```python
from build123d import *

# Parameters (mm, degrees)
BOSS_EXTRUDE1_DEPTH     = 5
CUT_EXTRUDE1_DEPTH      = 92.215662378
CUT_EXTRUDE1_DEPTH_BACK = 92.215662378
SKETCH2_R               = 2.75
CUT_EXTRUDE2_DEPTH      = 92.215662378
CUT_EXTRUDE2_DEPTH_BACK = 92.215662378
CHAMFER3_SIZE           = 2
CUT_EXTRUDE3_DEPTH      = 90.804241831
CUT_EXTRUDE3_DEPTH_BACK = 90.804241831
SKETCH4_W               = 120
SKETCH4_H               = 35
CHAMFER4_SIZE           = 2
SKETCH5_R               = 5
CUT_EXTRUDE4_DEPTH      = 3


with BuildPart() as part:
    # Sketch1 → Boss-Extrude1 (new body)
    with BuildSketch(Plane(origin=(0, 0, 0), x_dir=(1, 0, 0), z_dir=(0, 1, 0))):
        Polygon((-73.8, 35.677122405), (-83.8, 35.677122405), (-83.8, -35.677122405), (-73.8, -35.677122405), (73.8, -35.677122405), (83.8, -35.677122405), (83.8, 35.677122405), (73.8, 35.677122405), align=None)
    extrude(amount=BOSS_EXTRUDE1_DEPTH)

    # Sketch2 → Cut-Extrude1 (cut, two sides: drawn at the far end of the back side and taken through both)
    with BuildSketch(Plane(origin=(0, 5, 0), x_dir=(1, 0, 0), z_dir=(0, 1, 0)).offset(-CUT_EXTRUDE1_DEPTH_BACK)):
        with Locations(Location((-73.8, -15.5, 0), (0, 0, 270))):
            Circle(SKETCH2_R)
        with Locations(Location((-73.8, 15.5, 0), (0, 0, 270))):
            Circle(SKETCH2_R)
        with Locations(Location((73.797239672, -20, 0), (0, 0, 270))):
            Circle(SKETCH2_R)
        with Locations(Location((73.797239672, 20, 0), (0, 0, 270))):
            Circle(SKETCH2_R)
    extrude(amount=CUT_EXTRUDE1_DEPTH + CUT_EXTRUDE1_DEPTH_BACK, mode=Mode.SUBTRACT)

    # Sketch3 → Cut-Extrude2 (cut, two sides: drawn at the far end of the back side and taken through both)
    with BuildSketch(Plane(origin=(0, 5, 0), x_dir=(1, 0, 0), z_dir=(0, 1, 0)).offset(-CUT_EXTRUDE2_DEPTH_BACK)):
        Polygon((-63.8, -22.5), (53.754373535, -24.93027399), (90.089947098, -33.354383806), (45.106765394, -114.519737278), (-93.808894925, -48.481732373), (-93.808894925, -22.5), align=None)
        Polygon((53.754373535, 24.93027399), (-63.8, 22.5), (-93.808894925, 22.5), (-93.808894925, 75.103676807), (90.089947098, 109.537779365), (90.089947098, 33.354383806), align=None)
    extrude(amount=CUT_EXTRUDE2_DEPTH + CUT_EXTRUDE2_DEPTH_BACK, mode=Mode.SUBTRACT)

    # Chamfer3
    # the kernel refuses this chamfer: 2 mm, written as the material it takes off along each edge
    with BuildSketch(Plane(origin=(83.8, 0, 37.039476252), x_dir=(-0.9996219169112968, -0.027495876610586292, 0), z_dir=(0, 0, -1))) as chamfer3_piece_1:
        Polygon((CHAMFER3_SIZE * 0.999621916911, CHAMFER3_SIZE * 0.0274958766106), (-CHAMFER3_SIZE * 0.0274958766106, CHAMFER3_SIZE * 0.999621916911), (0, 0), align=None)
    extrude(amount=74.078952505, mode=Mode.SUBTRACT)
    with BuildSketch(Plane(origin=(58.89664073, 0, 25.036583248), x_dir=(0.020661384909083567, -0.027495876610586414, -0.9994083669566981), z_dir=(-0.9997863692752371, 0, -0.020669199583903272))) as chamfer3_piece_2_section:
        Polygon((CHAMFER3_SIZE * 0.999621916911, -CHAMFER3_SIZE * 0.0274958766106), (-CHAMFER3_SIZE * 0.0274958766106, -CHAMFER3_SIZE * 0.999621916911), (0, 0), align=None)
    chamfer3_piece_2 = extrude(amount=127.866224079, mode=Mode.PRIVATE)
    chamfer3_piece_2 = split(chamfer3_piece_2, bisect_by=Plane(origin=(6.389506061, 0.738517017, 22.5), z_dir=(0, 0, 1)), keep=Keep.TOP, mode=Mode.PRIVATE)
    chamfer3_piece_2 = split(chamfer3_piece_2, bisect_by=Plane(origin=(8.475011093, 0.738517017, 14.432618822), z_dir=(-0.22585154444898248, 0, 0.9741617318854243)), keep=Keep.TOP, mode=Mode.PRIVATE)
    add(chamfer3_piece_2, mode=Mode.SUBTRACT)
    with BuildSketch(Plane(origin=(-68.942267195, 0, -22.393690742), x_dir=(0.020661384909228912, -0.027495876610586358, 0.9994083669566951), z_dir=(0.9997863692752341, 0, -0.02066919958404867))) as chamfer3_piece_3_section:
        Polygon((CHAMFER3_SIZE * 0.999621916911, -CHAMFER3_SIZE * 0.0274958766106), (-CHAMFER3_SIZE * 0.0274958766106, -CHAMFER3_SIZE * 0.999621916911), (0, 0), align=None)
    chamfer3_piece_3 = extrude(amount=127.866224079, mode=Mode.PRIVATE)
    chamfer3_piece_3 = split(chamfer3_piece_3, bisect_by=Plane(origin=(6.389506061, 0.738517017, -22.5), z_dir=(0, 0, -1)), keep=Keep.TOP, mode=Mode.PRIVATE)
    chamfer3_piece_3 = split(chamfer3_piece_3, bisect_by=Plane(origin=(8.475011093, 0.738517017, -14.432618822), z_dir=(-0.22585154444898248, 0, -0.9741617318854243)), keep=Keep.TOP, mode=Mode.PRIVATE)
    add(chamfer3_piece_3, mode=Mode.SUBTRACT)

    # Sketch4 → Cut-Extrude3 (cut, two sides: drawn at the far end of the back side and taken through both)
    with BuildSketch(Plane.XZ.offset(-CUT_EXTRUDE3_DEPTH_BACK)):
        Rectangle(SKETCH4_W, SKETCH4_H)
    extrude(amount=CUT_EXTRUDE3_DEPTH + CUT_EXTRUDE3_DEPTH_BACK, mode=Mode.SUBTRACT)

    # Chamfer4
    chamfer4_edges = [part.edges().sort_by_distance(p)[0] for p in [
        (0, 0, -17.5),
        (60, 0, 0),
        (0, 0, 17.5),
        (-60, 0, 0),
    ]]
    chamfer(chamfer4_edges, length=CHAMFER4_SIZE)

    # Sketch5 → Cut-Extrude4 (cut)
    with BuildSketch(Plane.XZ):
        with Locations(Location((-73.8, 15.5, 0), (0, 0, 270))):
            Circle(SKETCH5_R)
        with Locations(Location((-73.8, -15.5, 0), (0, 0, 270))):
            Circle(SKETCH5_R)
        with Locations(Location((73.797239672, 20, 0), (0, 0, 270))):
            Circle(SKETCH5_R)
        with Locations(Location((73.797239672, -20, 0), (0, 0, 270))):
            Circle(SKETCH5_R)
    extrude(amount=-CUT_EXTRUDE4_DEPTH, mode=Mode.SUBTRACT)


solid = part.part
```
The model under review builds one solid part; all positions refer to its coordinate system, in mm. A direction names the side the tool comes from. Round coordinates to 2 decimals unless told otherwise and drop trailing zeros. Loops run counter-clockwise (first coordinate to the right, second up) from the corner with the lowest first, then second, coordinate; pieces in that order, holes last. Notation, with made-up numbers: M 1,19.25 L 25,19.25 A12 cw 25,32.25 Z; hole C 28.5,-8.75 d7. An arc over 180 degrees is marked long. Put each result on its own line as item: value.
Q1. Consider section A-A, the plane z = 4.5. Give the boundary of the cut face in (x, y).
Result set:
outline: M -83.8,0 L -62,0 L -60,2 L -60,5 L -83.8,5 Z; M 60,2 L 62,0 L 81.8,0 L 83.8,2 L 83.8,5 L 60,5 Z
Q2. Machinability: for faces 4 (the flat face through (-51, 1, -22.5)), 5 (the cylindrical face through (68.916, 1.479, -18.916)), 6 (the flat face through (60, 4, 0)), which of the approach directions +Z, -Z, +X, -X, +Y, -Y give a long, thin tool a straight path to every point of the face, cutting with its end or side? Answer none if there is none.
Result set:
face 4: -Z, -X, -Y
face 5: -Y
face 6: +Y, -Y
Q3. Consider section C-C, the plane x = -73.8. Give the boundary of the cut face in (y, z), then the cut area to 3 significant figures.
Result set:
outline: M 0,-22.5 L 5,-22.5 L 5,-18.25 L 3,-18.25 L 3,-20.5 L 0,-20.5 Z; M 0,-10.5 L 3,-10.5 L 3,-12.75 L 5,-12.75 L 5,12.75 L 3,12.75 L 3,10.5 L 0,10.5 Z; M 0,20.5 L 3,20.5 L 3,18.25 L 5,18.25 L 5,22.5 L 0,22.5 Z
area: 143 mm²
Q4. Consider section D-D, the plane x = -37. Give the boundary of the cut face in (y, z).
Result set:
outline: M 0,-22.5 L 1.45,-22.5 L 2,-23.05 L 5,-23.05 L 5,-17.5 L 2,-17.5 L 0,-19.5 Z; M 0,19.5 L 2,17.5 L 5,17.5 L 5,23.05 L 2,23.05 L 1.45,22.5 L 0,22.5 Z
Q5. To check wall thickness, follow L1, parallel to X at y = 3.15, z = -7; L2, parallel to Z at x = 73, y = 1.3; L3, parallel to X at y = 2.5, z = -16.5. State the ranges of each line that lie inside material, in increasing order.
Result set:
L1: x = -83.8 to -60, 60 to 83.8
L2: z = -29.39 to -24.94, -15.06 to 15.06, 24.94 to 29.39
L3: x = -83.8 to -78.7, -68.9 to -60, 60 to 70.23, 77.37 to 83.8
Q6. Consider section B-B, the plane x = -13. Give the boundary of the cut face in (y, z), then the cut area to 3 significant figures.
Result set:
outline: M 0,-22.5 L 0.95,-22.5 L 2,-23.55 L 5,-23.55 L 5,-17.5 L 2,-17.5 L 0,-19.5 Z; M 0,19.5 L 2,17.5 L 5,17.5 L 5,23.55 L 2,23.55 L 0.95,22.5 L 0,22.5 Z
area: 53.4 mm²
Q7. For pin 1 (3 mm diameter, centred on x = 74, z = -22.5, fed in from -Y); pin 2 (6 mm diameter, centred on x = 73.8, z = -20, fed in from +Y); pin 3 (1.5 mm diameter, centred on x = 26.5, y = 4, fed in from +Z); pin 4 (4.5 mm diameter, centred on x = -73.8, z = 15.5, fed in from +Y), all flat-tipped, find the tip position at first contact; note any pin that passes through.
Result set:
pin 1: stops at y = 3
pin 2: stops at y = 5
pin 3: stops at z = 24.38
pin 4: passes through
Q8. Mouldability with a two-part tool opening along X and no side actions: class faces 1 (the flat face through (-60, 4, 0)), 2 (the flat face through (83.8, 3, 0)), 3 (the flat face through (-1, 0, 21)) as released by +X, released by -X, zero draft, split by the parting line, or undercut.
Result set:
face 1: undercut
face 2: released by +X
face 3: zero draft
